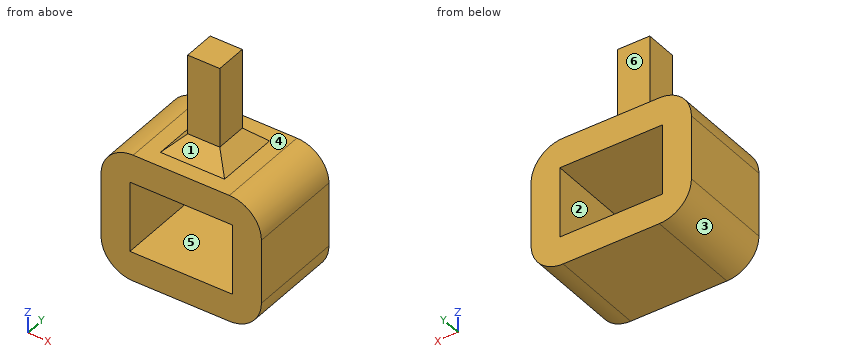
```python
from build123d import *

# Parameters (mm, degrees)
SKETCH1_W           = 50
SKETCH1_H           = 40
SKETCH1_W_2         = 32
SKETCH1_H_2         = 22
BOSS_EXTRUDE1_DEPTH = 30
SKETCH2_W           = 10
SKETCH2_H           = 10
BOSS_EXTRUDE2_DEPTH = 30
CHAMFER1_SIZE       = 5
FILLET1_R           = 10


with BuildPart() as part:
    # Sketch1 → Boss-Extrude1 (new body)
    with BuildSketch(Plane(origin=(0, 0, 0), x_dir=(1, 0, 0), z_dir=(0, 1, 0))):
        with Locations((1.8704784, -7.860892388)):
            Rectangle(SKETCH1_W, SKETCH1_H)
        with Locations((1.8704784, -7.860892388)):
            Rectangle(SKETCH1_W_2, SKETCH1_H_2, mode=Mode.SUBTRACT)
    extrude(amount=BOSS_EXTRUDE1_DEPTH)

    # Sketch2 → Boss-Extrude2 (add)
    with BuildSketch(Plane.XY.offset(27.860892388)):
        with Locations((1.8704784, 15)):
            Rectangle(SKETCH2_W, SKETCH2_H)
    extrude(amount=BOSS_EXTRUDE2_DEPTH)

    # Chamfer1
    chamfer1_edges = [part.edges().sort_by_distance(p)[0] for p in [
        (1.8704784, 10, 27.860892388),
        (6.8704784, 15, 27.860892388),
        (-3.1295216, 15, 27.860892388),
        (1.8704784, 20, 27.860892388),
    ]]
    chamfer(chamfer1_edges, length=CHAMFER1_SIZE)

    # Fillet1
    fillet1_edges = [part.edges().sort_by_distance(p)[0] for p in [
        (26.8704784, 15, 27.860892388),
        (-23.1295216, 15, 27.860892388),
        (-23.1295216, 15, -12.139107612),
        (26.8704784, 15, -12.139107612),
    ]]
    fillet(fillet1_edges, radius=FILLET1_R)


solid = part.part
```
Design review of the part built by this model. Coordinates are the model's own, in mm. Face numbers are marked on the shaded views. A direction names the side the tool comes from. Round coordinates to 2 decimals unless told otherwise and drop trailing zeros. Write each loop counter-clockwise with the first axis right and the second up, starting at its lowest first coordinate (ties: lowest second). Pieces come first, ordered by that corner, then holes.
Item 1: For probe 1 along X at (y, z) = (25, 10); probe 2 along Z at (x, y) = (-9.5, 27.75); probe 3 along Y at (x, z) = (0, 49), list the stretches that pass through material, from the lowest coordinate up.
Item 2: For the marked faces 4, 5 and 6, list the 3-axis set-ups (+Z, -Z, +X, -X, +Y, -Y) from which the entire face can be reached by the end or side of a thin tool; tool diameter is ignored.
Item 3: The part is to be moulded in two halves that separate along Z. For the marked faces 1, 2 and 3, say which applies: +Z half, -Z half, draft (parallel to the pull), parting line (faces both ways), or undercut.
Item 4: We need section C-C on x = -12. Write out the cut boundary in (y, z).
Item 5: We need section A-A on x = 4. Write out the cut boundary in (y, z).
Item 6: We need section D-D on y = 15.25. Write out the cut boundary in (x, z), and give its area (3 significant figures).
Item 7: We need section B-B on y = 27.5. Write out the cut boundary in (x, z), and give its area (3 significant figures).
Item 8: Clearance check with flat-ended pins moving along their axes: pin 1 Ø1 at (x, y) = (11, 15) entering from +Z; pin 2 Ø10 at (x, y) = (17.5, 8.5) entering from +Z; pin 3 Ø3 at (y, z) = (16, 39.5) entering from +X. State where each tip first meets the part, or that it passes through.
Returned:
1. probe 1: x = -23.13 to -14.13, 17.87 to 26.87
1. probe 2: z = -12.14 to -3.14, 18.86 to 27.86
1. probe 3: y = 10 to 20
2. face 4: +Z
2. face 5: +Y, -Y
2. face 6: +Z, +X, -X, +Y
3. face 1: +Z half
3. face 2: undercut
3. face 3: -Z half
4. outline: (0, -12.14) - (30, -12.14) - (30, -3.14) - (0, -3.14) - close; (0, 18.86) - (30, 18.86) - (30, 27.86) - (0, 27.86) - close
5. outline: (0, -12.14) - (30, -12.14) - (30, -3.14) - (0, -3.14) - close; (0, 18.86) - (30, 18.86) - (30, 27.86) - (25, 27.86) - (20, 32.86) - (20, 57.86) - (10, 57.86) - (10, 32.86) - (5, 27.86) - (0, 27.86) - close
6. outline: (-23.13, -2.14) arc R10 ccw to (-13.13, -12.14) - (16.87, -12.14) arc R10 ccw to (26.87, -2.14) - (26.87, 17.86) arc R10 ccw to (16.87, 27.86) - (11.87, 27.86) - (6.87, 32.86) - (6.87, 57.86) - (-3.13, 57.86) - (-3.13, 32.86) - (-8.13, 27.86) - (-13.13, 27.86) arc R10 ccw to (-23.13, 17.86) - close; hole (-14.13, -3.14) - (17.87, -3.14) - (17.87, 18.86) - (-14.13, 18.86) - close
6. area: 1,540 mm2
7. outline: (-23.13, -2.14) arc R10 ccw to (-13.13, -12.14) - (16.87, -12.14) arc R10 ccw to (26.87, -2.14) - (26.87, 17.86) arc R10 ccw to (16.87, 27.86) - (-13.13, 27.86) arc R10 ccw to (-23.13, 17.86) - close; hole (-14.13, -3.14) - (17.87, -3.14) - (17.87, 18.86) - (-14.13, 18.86) - close
7. area: 1,210 mm2
8. pin 1: stops at z = 29.23
8. pin 2: stops at z = 27.86
8. pin 3: stops at x = 6.87
